The figure shows three views and two pictorial views of one solid part (mm, origin at its lowest corner). Answer the questions. A direction names the side the tool comes from. Coordinates: 2 decimals unless noted, no trailing zeros. Write each loop counter-clockwise with the first axis right and the second up, starting at its lowest first coordinate (ties: lowest second). Pieces come first, ordered by that corner, then holes. Notation, with made-up numbers: M -19.5,77 L -2.5,77 A18 ccw -2.5,85 Z; hole C -14.5,3 d10. An arc over 180 degrees is marked long. Use CSV: the item, a comma, the result in double quotes.
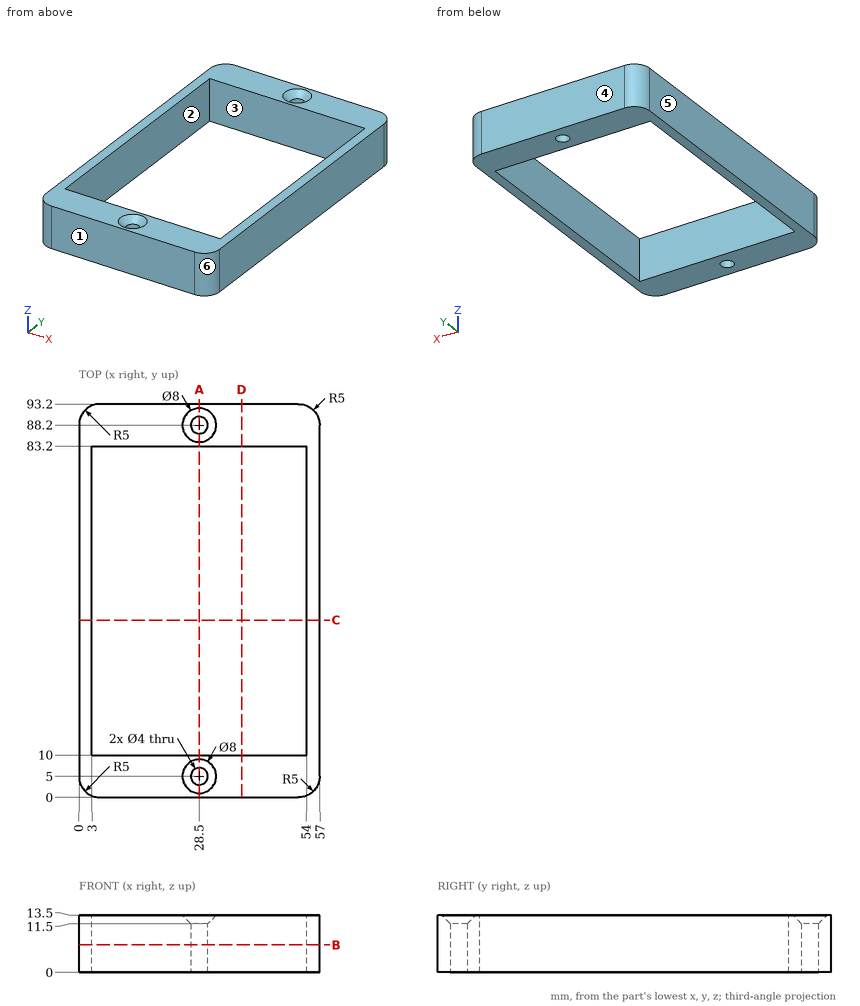
Item 1: Given pin 1 (3.5 mm diameter, centred on x = 28.5, y = 5, fed in from -Z), flat-ended and moving along its own axis, determine where the tip first touches the part or whether it passes through.
Answer:
pin 1,"passes through"
Item 2: The part is cut by section A-A (x = 28.5). Write down the section's boundary in (y, z), then the cut area to 3 significant figures.
Answer:
outline,"M 0,0 L 3,0 L 3,11.5 L 1,13.5 L 0,13.5 Z; M 7,0 L 10,0 L 10,13.5 L 9,13.5 L 7,11.5 Z; M 83.2,0 L 86.2,0 L 86.2,11.5 L 84.2,13.5 L 83.2,13.5 Z; M 90.2,0 L 93.2,0 L 93.2,13.5 L 92.2,13.5 L 90.2,11.5 Z"
area,"154 mm2"
Item 3: The part is cut by section C-C (y = 42). Write down the section's boundary in (x, z).
Answer:
outline,"M 0,0 L 3,0 L 3,13.5 L 0,13.5 Z; M 54,0 L 57,0 L 57,13.5 L 54,13.5 Z"
Item 4: The part is cut by section B-B (z = 6.5). Write down the section's boundary in (x, y), then the cut area to 3 significant figures.
Answer:
outline,"M 0,5 A5 ccw 5,0 L 52,0 A5 ccw 57,5 L 57,88.2 A5 ccw 52,93.2 L 5,93.2 A5 ccw 0,88.2 Z; hole M 3,10 L 54,10 L 54,83.2 L 3,83.2 Z; hole C 28.5,5 d4; hole C 28.5,88.2 d4"
area,"1,530 mm2"
Item 5: The part is cut by section D-D (x = 38.5). Write down the section's boundary in (y, z), then the cut area to 3 significant figures.
Answer:
outline,"M 0,0 L 10,0 L 10,13.5 L 0,13.5 Z; M 83.2,0 L 93.2,0 L 93.2,13.5 L 83.2,13.5 Z"
area,"270 mm2"
Item 6: Consider probe 1 along Y at (x, z) = (39, 10); probe 2 along Y at (x, z) = (28.5, 6.75); probe 3 along X at (y, z) = (38, 12). Determine where each line is inside the solid, lowest interval first.
Answer:
probe 1,"y = 0 to 10, 83.2 to 93.2"
probe 2,"y = 0 to 3, 7 to 10, 83.2 to 86.2, 90.2 to 93.2"
probe 3,"x = 0 to 3, 54 to 57"
Item 7: For a pull along Y with two mould halves and no side action, classify the marked faces 3, 4, 5 and 6 as released by +Y, released by -Y, zero draft, split by the parting line, or undercut.
Answer:
face 3,"undercut"
face 4,"released by +Y"
face 5,"zero draft"
face 6,"released by -Y"
Item 8: A tool of negligible diameter and unlimited length cuts with its end or side. For the marked faces 1 and 2, from which of +Z, -Z, +X, -X, +Y, -Y can it reach the whole face along a straight path? Write none if from no direction.
Answer:
face 1,"+Z, -Z, +X, -X, -Y"
face 2,"+Z, -Z"
